```python
from build123d import *
from OCP.BRepFilletAPI import BRepFilletAPI_MakeChamfer

# Parameters (mm, degrees)
SKETCH_1_R                            = 51.8
SKETCH_1_R_2                          = 48.6
EXTRUDE_1_DEPTH                       = 10
EXTRUDE_START                         = 43.299942
EXTRUDE_4_DEPTH                       = 5.300058
CHAMFER_1_SIZE                        = 5
CHAMFER_1_SIZE2                       = 3.767770251
PATTERN_CIRCULAR_4_COUNT              = 4
CHAMFER_1_OF_PATTERN_CIRCULAR_4_SIZE  = 5
CHAMFER_1_OF_PATTERN_CIRCULAR_4_SIZE2 = 3.767770251


with BuildPart() as part:
    # 草图1 → 凸台-拉伸1 (new body)
    with BuildSketch(Plane(origin=(0, 0, 0), x_dir=(1, 0, 0), z_dir=(0, 1, 0))):
        with Locations(Location((0, 0, 0), (0, 0, 90))):
            Circle(SKETCH_1_R)
        with Locations(Location((0, 0, 0), (0, 0, 90))):
            Circle(SKETCH_1_R_2, mode=Mode.SUBTRACT)
    extrude(amount=EXTRUDE_1_DEPTH)

    # 草图2 → 凸台-拉伸4 (add)
    with BuildSketch(Plane.XY.offset(EXTRUDE_START)):
        with BuildLine():
            Line((4, 2.6), (4, 0))
            Line((4, 0), (-4, 0))
            Line((-4, 0), (-4, 2.6))
            ThreePointArc((-4, 2.6), (0, 6.6), (4, 2.6))
        make_face()
    extrude_4 = extrude(amount=EXTRUDE_4_DEPTH)

    # 倒角1: one chamfer whose edges measure the first distance from different faces: ONE call of the kernel's chamfer builder (chamfer() names one face for all edges)
    chamfer_1_edges_1 = [part.edges().sort_by_distance(p)[0] for p in [
        (0, 6.6, 43.299942),
    ]]
    chamfer_1_side_1 = [part.faces().sort_by_distance(p)[0] for p in [
        (0, 6.6, 45.95017715),
    ]]
    chamfer_1_edges_2 = [part.edges().sort_by_distance(p)[0] for p in [
        (4, 1.3, 43.299942),
    ]]
    chamfer_1_side_2 = [part.faces().sort_by_distance(p)[0] for p in [
        (4, 1.3, 45.867526616),
    ]]
    chamfer_1 = BRepFilletAPI_MakeChamfer(part.part.solid().wrapped)
    for e in chamfer_1_edges_1:
        chamfer_1.Add(CHAMFER_1_SIZE, CHAMFER_1_SIZE2, e.wrapped, chamfer_1_side_1[0].wrapped)  # the first distance lies on this face
    for e in chamfer_1_edges_2:
        chamfer_1.Add(CHAMFER_1_SIZE, CHAMFER_1_SIZE2, e.wrapped, chamfer_1_side_2[0].wrapped)  # the first distance lies on this face
    add(Compound.cast(chamfer_1.Shape()), mode=Mode.REPLACE)

    # 阵列(圆周)4: 凸台-拉伸4 ×4 about axis
    pattern_circular_4_axis = Axis((0, 0, 0), (0, 1, 0))
    for i in range(1, PATTERN_CIRCULAR_4_COUNT):
        add(extrude_4.rotate(pattern_circular_4_axis, i * 360 / PATTERN_CIRCULAR_4_COUNT))

    # 倒角1 of 阵列(圆周)4: one chamfer whose edges measure the first distance from different faces: ONE call of the kernel's chamfer builder (chamfer() names one face for all edges)
    chamfer_1_of_pattern_circular_4_edges_1 = [part.edges().sort_by_distance(p)[0] for p in [
        (43.299942, 6.6, 0),
    ]]
    chamfer_1_of_pattern_circular_4_side_1 = [part.faces().sort_by_distance(p)[0] for p in [
        (45.95017715, 6.6, 0),
    ]]
    chamfer_1_of_pattern_circular_4_edges_2 = [part.edges().sort_by_distance(p)[0] for p in [
        (43.299942, 1.3, -4),
    ]]
    chamfer_1_of_pattern_circular_4_side_2 = [part.faces().sort_by_distance(p)[0] for p in [
        (45.867526616, 1.3, -4),
    ]]
    chamfer_1_of_pattern_circular_4_edges_3 = [part.edges().sort_by_distance(p)[0] for p in [
        (0, 6.6, -43.299942),
    ]]
    chamfer_1_of_pattern_circular_4_side_3 = [part.faces().sort_by_distance(p)[0] for p in [
        (0, 6.6, -45.95017715),
    ]]
    chamfer_1_of_pattern_circular_4_edges_4 = [part.edges().sort_by_distance(p)[0] for p in [
        (-4, 1.3, -43.299942),
    ]]
    chamfer_1_of_pattern_circular_4_side_4 = [part.faces().sort_by_distance(p)[0] for p in [
        (-4, 1.3, -45.867526616),
    ]]
    chamfer_1_of_pattern_circular_4_edges_5 = [part.edges().sort_by_distance(p)[0] for p in [
        (-43.299942, 6.6, 0),
    ]]
    chamfer_1_of_pattern_circular_4_side_5 = [part.faces().sort_by_distance(p)[0] for p in [
        (-45.95017715, 6.6, 0),
    ]]
    chamfer_1_of_pattern_circular_4_edges_6 = [part.edges().sort_by_distance(p)[0] for p in [
        (-43.299942, 1.3, 4),
    ]]
    chamfer_1_of_pattern_circular_4_side_6 = [part.faces().sort_by_distance(p)[0] for p in [
        (-45.867526616, 1.3, 4),
    ]]
    chamfer_1_of_pattern_circular_4 = BRepFilletAPI_MakeChamfer(part.part.solid().wrapped)
    for e in chamfer_1_of_pattern_circular_4_edges_1:
        chamfer_1_of_pattern_circular_4.Add(CHAMFER_1_OF_PATTERN_CIRCULAR_4_SIZE, CHAMFER_1_OF_PATTERN_CIRCULAR_4_SIZE2, e.wrapped, chamfer_1_of_pattern_circular_4_side_1[0].wrapped)  # the first distance lies on this face
    for e in chamfer_1_of_pattern_circular_4_edges_2:
        chamfer_1_of_pattern_circular_4.Add(CHAMFER_1_OF_PATTERN_CIRCULAR_4_SIZE, CHAMFER_1_OF_PATTERN_CIRCULAR_4_SIZE2, e.wrapped, chamfer_1_of_pattern_circular_4_side_2[0].wrapped)  # the first distance lies on this face
    for e in chamfer_1_of_pattern_circular_4_edges_3:
        chamfer_1_of_pattern_circular_4.Add(CHAMFER_1_OF_PATTERN_CIRCULAR_4_SIZE, CHAMFER_1_OF_PATTERN_CIRCULAR_4_SIZE2, e.wrapped, chamfer_1_of_pattern_circular_4_side_3[0].wrapped)  # the first distance lies on this face
    for e in chamfer_1_of_pattern_circular_4_edges_4:
        chamfer_1_of_pattern_circular_4.Add(CHAMFER_1_OF_PATTERN_CIRCULAR_4_SIZE, CHAMFER_1_OF_PATTERN_CIRCULAR_4_SIZE2, e.wrapped, chamfer_1_of_pattern_circular_4_side_4[0].wrapped)  # the first distance lies on this face
    for e in chamfer_1_of_pattern_circular_4_edges_5:
        chamfer_1_of_pattern_circular_4.Add(CHAMFER_1_OF_PATTERN_CIRCULAR_4_SIZE, CHAMFER_1_OF_PATTERN_CIRCULAR_4_SIZE2, e.wrapped, chamfer_1_of_pattern_circular_4_side_5[0].wrapped)  # the first distance lies on this face
    for e in chamfer_1_of_pattern_circular_4_edges_6:
        chamfer_1_of_pattern_circular_4.Add(CHAMFER_1_OF_PATTERN_CIRCULAR_4_SIZE, CHAMFER_1_OF_PATTERN_CIRCULAR_4_SIZE2, e.wrapped, chamfer_1_of_pattern_circular_4_side_6[0].wrapped)  # the first distance lies on this face
    add(Compound.cast(chamfer_1_of_pattern_circular_4.Shape()), mode=Mode.REPLACE)


solid = part.part
```
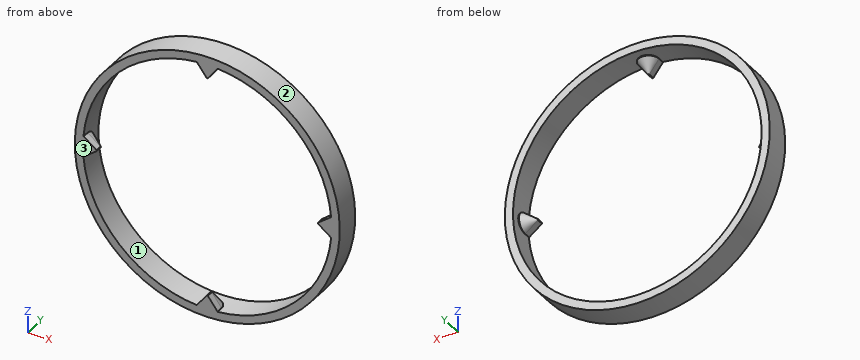
Can you work these out from the model? Positions are in its coordinate system, mm. Face numbers are marked on the shaded views. Give positions to 0.01 mm unless a question says otherwise; leave off trailing zeros. Order: outer loops, then holes, each group sorted by start corner. A loop starts at its lowest first (then second) coordinate and runs counter-clockwise, first axis right, second up. Notation, with made-up numbers: (-0.75, -28.5) - (35.25, -28.5) arc R25 cw to (35.25, 9.5) - close; hole circle Ø3 at (48, -13). An arc over 180 degrees is marked (long way). Use a Markdown table: item, result. Add a question column.
Q1. I'm going to push flat-ended pins straight in: pin 1 (0.5 mm diameter, centred on y = 1, z = 0, fed in from -X); pin 2 (6 mm diameter, centred on y = 3.5, z = 17, fed in from -X); pin 3 (2 mm diameter, centred on y = 7.5, z = -33, fed in from -X). Where does each tip first touch, or does it pass through?
Q2. If we section it at B-B on x = 28: Write out the boundary of the cut face in (y, z), plus the area to 3 significant figures.
Q3. If we section it at A-A on z = 27.5: Write out the boundary of the cut face in (x, y).
Q4. If we mould it in two halves opening along X, with no side actions, what happens to the marked faces 1, 2 and 3? For each: released by +X, released by -X, zero draft, split by the parting line, or undercut.
Q5. Please list where these lines run through material, in increasing order: line 1 along X through (y, z) = (2.5, 0); line 2 along X through (y, z) = (7, 0); line 3 along Z through (x, y) = (42, 5.5).
Answers follow:
| question | item | result |
|---|---|---|
| 1 | pin 1 | stops at x = -51.8 |
| 1 | pin 2 | stops at x = -49.87 |
| 1 | pin 3 | stops at x = -40.73 |
| 2 | outline | (0, -43.58) - (10, -43.58) - (10, -39.72) - (0, -39.72) - close; (0, 39.72) - (10, 39.72) - (10, 43.58) - (0, 43.58) - close |
| 2 | area | 77.1 mm^2 |
| 3 | outline | (-43.9, 0) - (-40.07, 0) - (-40.07, 10) - (-43.9, 10) - close; (40.07, 0) - (43.9, 0) - (43.9, 10) - (40.07, 10) - close |
| 4 | face 1 | undercut |
| 4 | face 2 | split by the parting line |
| 4 | face 3 | zero draft |
| 5 | line 1 | x = -51.8 to -43.3, 43.3 to 51.8 |
| 5 | line 2 | x = -51.8 to -48.6, 48.6 to 51.8 |
| 5 | line 3 | z = -30.32 to -24.45, 24.45 to 30.32 |
